from build123d import *

# Parameters (mm, degrees)
BOSS_EXTRUDE1_DEPTH = 11.5
SHELL1_T            = -3
SKETCH3_R           = 1.3
CUT_EXTRUDE1_DEPTH  = 94
SKETCH4_R           = 1.3
CUT_EXTRUDE2_DEPTH  = 94
FILLET1_R           = 2
CUT_EXTRUDE3_DEPTH  = 79
CUT_EXTRUDE4_DEPTH  = 79
FILLET2_R           = 2
SKETCH7_R           = 1.6
CUT_EXTRUDE5_DEPTH  = 10
SKETCH8_R           = 1
CUT_EXTRUDE7_DEPTH  = 79
CUT_EXTRUDE8_DEPTH  = 1.5
CUT_EXTRUDE9_DEPTH  = 1.5
FILLET3_R           = 1


with BuildPart() as part:
    # Sketch1 → Boss-Extrude1 (new body)
    with BuildSketch(Plane(origin=(0, 0, 0), x_dir=(1, 0, 0), z_dir=(0, 1, 0))):
        Polygon((-11.213203436, 40), (18.786796564, 40), (40, 18.786796564), (40, -11.213203436), (18.786796564, -32.426406871), (-11.213203436, -32.426406871), (-32.426406871, -11.213203436), (-32.426406871, 18.786796564), align=None)
    extrude(amount=BOSS_EXTRUDE1_DEPTH)

    # Shell1
    shell1_openings = [part.faces().sort_by_distance(p)[0] for p in [
        (3.786796564, 11.5, -3.786796564),
    ]]
    offset(amount=SHELL1_T, openings=shell1_openings, kind=Kind.INTERSECTION)

    # Sketch3 → Cut-Extrude1 (cut)
    with BuildSketch(Plane(origin=(-21.819805153, 0, 21.819805153), x_dir=(0.7071067811865558, 0, 0.7071067811865392), z_dir=(-0.7071067811865392, 0, 0.7071067811865558))):
        with Locations((-9, 7.25)):
            Circle(SKETCH3_R)
        with Locations((9, 7.25)):
            Circle(SKETCH3_R)
    extrude(amount=-CUT_EXTRUDE1_DEPTH, mode=Mode.SUBTRACT)

    # Sketch4 → Cut-Extrude2 (cut)
    with BuildSketch(Plane(origin=(-25.606601718, 0, -25.606601718), x_dir=(-0.7071067811865556, 0, 0.7071067811865396), z_dir=(-0.7071067811865396, 0, -0.7071067811865556))):
        with Locations((-14.355339059, 7.25)):
            Circle(SKETCH4_R)
        with Locations((3.644660941, 7.25)):
            Circle(SKETCH4_R)
    extrude(amount=-CUT_EXTRUDE2_DEPTH, mode=Mode.SUBTRACT)

    # Fillet1
    fillet1_edges = [part.edges().sort_by_distance(p)[0] for p in [
        (40, 5.75, -18.786796564),
        (40, 5.75, 11.213203436),
        (18.786796564, 5.75, 32.426406871),
        (-11.213203436, 5.75, 32.426406871),
        (-32.426406871, 5.75, 11.213203436),
        (-32.426406871, 5.75, -18.786796564),
        (-11.213203436, 5.75, -40),
        (18.786796564, 5.75, -40),
    ]]
    fillet(fillet1_edges, radius=FILLET1_R)

    # Sketch5 → Cut-Extrude3 (cut)
    with BuildSketch(Plane.XY.offset(32.426406871)):
        Polygon((3.786796564, 7), (13.286796564, 7), (13.286796564, 11.5), (-5.713203436, 11.5), (-5.713203436, 7), align=None)
    extrude(amount=-CUT_EXTRUDE3_DEPTH, mode=Mode.SUBTRACT)

    # Sketch6 → Cut-Extrude4 (cut)
    with BuildSketch(Plane.ZY.offset(32.426406871)):
        Polygon((-3.786796564, 7), (5.713203436, 7), (5.713203436, 11.5), (-13.286796564, 11.5), (-13.286796564, 7), align=None)
    extrude(amount=-CUT_EXTRUDE4_DEPTH, mode=Mode.SUBTRACT)

    # Fillet2
    fillet2_edges = [part.edges().sort_by_distance(p)[0] for p in [
        (-5.713203436, 7, -38.5),
        (-5.713203436, 11.5, -38.5),
        (13.286796564, 11.5, -38.5),
        (13.286796564, 7, -38.5),
        (-5.713203436, 7, 30.926406871),
        (-5.713203436, 11.5, 30.926406871),
        (13.286796564, 11.5, 30.926406871),
        (13.286796564, 7, 30.926406871),
        (38.5, 7, -13.286796564),
        (-30.926406871, 7, -13.286796564),
        (38.5, 11.5, -13.286796564),
        (-30.926406871, 11.5, -13.286796564),
        (38.5, 11.5, 5.713203436),
        (-30.926406871, 11.5, 5.713203436),
        (38.5, 7, 5.713203436),
        (-30.926406871, 7, 5.713203436),
    ]]
    fillet(fillet2_edges, radius=FILLET2_R)

    # Sketch7 → Cut-Extrude5 (cut)
    with BuildSketch(Plane(origin=(0, 0, 0), x_dir=(-1, 0, 0), z_dir=(0, -1, 0))):
        with Locations(Location((6.213203436, -6.213203436, 0), (0, 0, 90))):
            Circle(SKETCH7_R)
        with Locations(Location((-13.786796564, -6.213203436, 0), (0, 0, 90))):
            Circle(SKETCH7_R)
        with Locations(Location((-13.786796564, 13.786796564, 0), (0, 0, 90))):
            Circle(SKETCH7_R)
        with Locations(Location((6.213203436, 13.786796564, 0), (0, 0, 90))):
            Circle(SKETCH7_R)
    extrude(amount=-CUT_EXTRUDE5_DEPTH, mode=Mode.SUBTRACT)

    # Sketch8 → Cut-Extrude7 (cut)
    with BuildSketch(Plane(origin=(40, 0, 0), x_dir=(0, 0, -1), z_dir=(1, 0, 0))):
        with Locations((-8.213203436, 10)):
            Circle(SKETCH8_R)
        with Locations((-8.213203436, 3)):
            Circle(SKETCH8_R)
        with Locations((15.786796564, 3)):
            Circle(SKETCH8_R)
        with Locations(Location((15.786796564, 10, 0), (0, 0, 180))):
            Circle(SKETCH8_R)
    extrude(amount=-CUT_EXTRUDE7_DEPTH, mode=Mode.SUBTRACT)

    # Sketch10 → Cut-Extrude8 (cut)
    with BuildSketch(Plane(origin=(0, 3, 0), x_dir=(1, 0, 0), z_dir=(0, 1, 0))):
        Polygon((17.544155877, 37), (37, 17.544155877), (37, -9.970562748), (17.544155877, -29.426406871), (-9.970562748, -29.426406871), (-29.426406871, -9.970562748), (-29.426406871, 17.544155877), (-9.970562748, 37), align=None)
    extrude(amount=-CUT_EXTRUDE8_DEPTH, mode=Mode.SUBTRACT)

    # Sketch12 → Cut-Extrude9 (cut)
    with BuildSketch(Plane(origin=(0, 1.5, 0), x_dir=(1, 0, 0), z_dir=(0, 1, 0))):
        Polygon((-26.426406871, 20.544155877), (-29.426406871, 17.544155877), (-29.426406871, 12.286796564), (-26.426406871, 12.286796564), align=None)
        Polygon((-26.426406871, -4.713203436), (-29.426406871, -4.713203436), (-29.426406871, -9.970562748), (-26.426406871, -12.970562748), align=None)
        Polygon((34, 12.286796564), (37, 12.286796564), (37, 17.544155877), (34, 20.544155877), align=None)
        Polygon((37, -9.970562748), (37, -4.713203436), (34, -4.713203436), (34, -12.970562748), align=None)
    extrude(amount=-CUT_EXTRUDE9_DEPTH, mode=Mode.SUBTRACT)

    # Fillet3
    fillet3_edges = [part.edges().sort_by_distance(p)[0] for p in [
        (-26.426406871, 0.75, 4.713203436),
        (-26.426406871, 0.75, 12.970562748),
        (-29.426406871, 0.75, 4.713203436),
        (34, 0.75, -12.286796564),
        (34, 0.75, -20.544155877),
        (37, 0.75, -12.286796564),
        (37, 0.75, 4.713203436),
        (34, 0.75, 12.970562748),
        (34, 0.75, 4.713203436),
        (-29.426406871, 0.75, -12.286796564),
        (-26.426406871, 0.75, -20.544155877),
        (-26.426406871, 0.75, -12.286796564),
    ]]
    fillet(fillet3_edges, radius=FILLET3_R)


solid = part.part
Read the model definition and answer for the solid it produces. Units are mm, in the model's axes. A direction names the side the tool comes from. Give positions to 0.01 mm unless a question says otherwise; leave off trailing zeros. Write each loop counter-clockwise with the first axis right and the second up, starting at its lowest first coordinate (ties: lowest second). Pieces come first, ordered by that corner, then holes. Notation, with made-up numbers: (82, 72) -> (108, 72) arc R24 ccw to (108, 82) -> close; hole circle Ø1 at (11, 15). An arc over 180 degrees is marked (long way). Answer as a JSON object with one key per item and string values. Group by question number.
1) Consider L1, parallel to Z at x = -30.4, y = 3; L2, parallel to Z at x = 14.5, y = 5.5; L3, parallel to X at y = 3, z = 3. Determine where each line is inside the solid, lowest interval first. Write a range as from..to.
2) A tool of negligible diameter and unlimited length cuts with its end or side. For faces 1 (the cylindrical face through (-5.14, 7.6, 30.91)), 2 (the cylindrical face through (38.521, 10.93, 6.315)), 3 (the flat face through (37, 4, -4)), from which of +Z, -Z, +X, -X, +Y, -Y can it reach the whole face along a straight path? Write none if from no direction.
3) Find section B-B (x = 29). Write down the section's boundary in (y, z).
4) Each of these flat-tipped pins is pushed along its axis until it touches: P1, Ø6, axis at y = 3, z = 13.5, coming from the +X side; P2, Ø1.2, axis at y = 10, z = 8.21, coming from the +X side; P3, Ø1.1, axis at x = 35.5, y = 0.5, coming from the +Z side; P4, Ø4, axis at x = 23.5, y = 6, coming from the +Z side. Where does it stop, or does it pass through?
5) Find section A-A (z = 22). Write down the section's boundary in (x, y), and give its area (3 significant figures).
6) The mould has two halves that part along X. Classify faces 4 (the flat face through (-21, 11.5, -29)), 5 (the cylindrical face through (12.716, 7.601, -38.521)), 6 (the flat face through (40, 4, -4)): +X half, -X half, draft (parallel to the pull), parting line (faces both ways), or undercut.
Values follow:
{
 "1": {"L1": "z = -20.81..-16.79, -14.79..7.21, 9.21..13.24", "L2": "z = -40..-37, 29.43..32.43", "L3": "x = -32.43..-29.43, 37..40"},
 "2": {"face 1": "+Z, -Z, +Y", "face 2": "+X, -X, +Y", "face 3": "+Y"},
 "3": {"outline": "(0, -29.79) -> (11.5, -29.79) -> (11.5, -25.54) -> (1.5, -25.54) -> (1.5, 17.97) -> (11.5, 17.97) -> (11.5, 22.21) -> (0, 22.21) -> close"},
 "4": {"P1": "stops at x = 40", "P2": "passes through", "P3": "stops at z = 16.26", "P4": "stops at z = 29.71"},
 "5": {"outline": "(-21.64, 0) -> (29.21, 0) -> (29.21, 11.5) -> (24.97, 11.5) -> (24.97, 1.5) -> (-17.4, 1.5) -> (-17.4, 11.5) -> (-21.64, 11.5) -> close", "area": "161 mm2"},
 "6": {"face 4": "draft", "face 5": "undercut", "face 6": "+X half"}
}
